from build123d import *

# Parameters (mm, degrees)
F3_W     = 1.5875
F3_H     = 15.875
F2_DEPTH = 2.38125


with BuildPart() as f1:
    # F0 (on Front) → F1 (revolve)
    with BuildSketch(Plane.XZ):
        Polygon((-9.525, 7.9375), (-15.875, 7.9375), (-15.875, 0), (15.875, 0), (15.875, 4.45897), (14.77772, 5.55625), (-6.35, 5.55625), (-6.35, 4.45897), (-9.525, 4.45897), align=None)
    revolve(axis=Axis((0, 0, 0), (1, 0, 0)))

    # F3 (on face) → F2 (cut)
    with BuildSketch(Plane(origin=(-15.875, 0, 0), x_dir=(0, -1, 0), z_dir=(-1, 0, 0))):
        Rectangle(F3_W, F3_H)
    extrude(amount=-F2_DEPTH, mode=Mode.SUBTRACT)


solid = f1.part
Verification items for the finished model (mm, model axes). A direction names the side the tool comes from. Give positions to 0.01 mm unless a question says otherwise; leave off trailing zeros. Write each loop counter-clockwise with the first axis right and the second up, starting at its lowest first coordinate (ties: lowest second). Pieces come first, ordered by that corner, then holes. Notation, with made-up numbers: (20, -6.75) - (76, -6.75) arc R15 cw to (76, 15.25) - close; hole circle Ø7 at (69.5, -27). An arc over 180 degrees is marked (long way). Answer as CSV lines item,"result". Start each with the question number.
1. Draft check along X on faces 5 (the face through (-9.525, 3.4, -3.4)), 6 (the face through (-13.494, 0, 0)), 7 (the face through (-15, -0.794, 0)). Enter one of: pulls with the +X half, pulls with the -X half, needs draft (parallel to the pull), parting line crosses it, or undercut.
2. Sectioned sample at C-C (x = -7). Record the boundary of the cut face in (y, z).
3. Depth check by flat-ended pin: pin 1 (1.9 mm diameter, centred on x = -14, z = 2.5, fed in from +Y); pin 2 (1 mm diameter, centred on x = 10, z = -1, fed in from +Y); pin 3 (1.3 mm diameter, centred on y = 0, z = -3, fed in from -X). Enter the tip coordinate at first touch or a pass-through.
4. Sectioned sample at D-D (x = -10.5). Record the boundary of the cut face in (y, z) (1 decimal).
5. Thickness scan on line 1 (Z direction, x = -8, y = 0); line 2 (X direction, y = 0.25, z = 1.5) (3 decimals); line 3 (X direction, y = 5, z = 6) (3 decimals). Record the ranges inside material, lowest first.
6. Set-up check for faces 1 (the face through (4.07, -1.67, 5.3)), 2 (the face through (-15, 0.794, 0)), 3 (the face through (-6.35, -5, 0)), 4 (the face through (-15.875, 4, 0)): record each of +Z, -Z, +X, -X, +Y, -Y from which the full face is reachable in a straight line by a thin tool's end or side.
Derived:
1,face 5,"undercut"
1,face 6,"pulls with the -X half"
1,face 7,"needs draft"
2,outline,"circle Ø8.92 at (0, 0)"
3,pin 1,"y = 7.78"
3,pin 2,"y = 5.53"
3,pin 3,"x = -13.49"
4,outline,"circle Ø15.9 at (0, 0)"
5,line 1,"-4.46 to 4.46"
5,line 2,"-13.494 to 15.875"
5,line 3,"-15.875 to -9.525"
6,face 1,"+X"
6,face 2,"+Z, -Z, -X"
6,face 3,"none"
6,face 4,"+Z, -Z, -X, +Y, -Y"
